```python
from build123d import *

# Parameters (mm, degrees)
SKETCH_1_W          = 55.5
SKETCH_1_H          = 46.5
EXTRUDE_1_DEPTH     = 15
SKETCH_2_W          = 6.5
SKETCH_2_H          = 6.5
CUT_EXTRUDE_1_DEPTH = 14
FILLET_1_R          = 2
SKETCH_3_W          = 4
SKETCH_3_H          = 34
EXTRUDE_2_DEPTH     = 5
SKETCH_4_W          = 55.5
SKETCH_4_H          = 46.5
EXTRUDE_3_DEPTH     = 1.5
SKETCH_5_R          = 1.5
CUT_EXTRUDE_2_DEPTH = 1
SKETCH_6_R          = 1.75
CUT_EXTRUDE_3_DEPTH = 2
SKETCH_7_W          = 33.995169083
SKETCH_7_H          = 13.97859025
SKETCH_7_W_2        = 5.219477383
SKETCH_7_H_2        = 24.424681599
SKETCH_7_W_3        = 25.720685112
SKETCH_7_H_3        = 6.003184014
EXTRUDE_4_DEPTH     = 10
SKETCH_8_W          = 33.995169083
SKETCH_8_H          = 13.97859025
SKETCH_8_W_2        = 25.720685112
SKETCH_8_H_2        = 6.003184014
CUT_EXTRUDE_4_DEPTH = 3
SKETCH_10_W         = 5.219477383
SKETCH_10_H         = 24.424681599
EXTRUDE_6_DEPTH     = 1.5


with BuildPart() as part:
    # 草图1 → 凸台-拉伸1 (new body)
    with BuildSketch(Plane.XY):
        Rectangle(SKETCH_1_W, SKETCH_1_H)
    extrude(amount=EXTRUDE_1_DEPTH)

    # 草图2 → 切除-拉伸1 (cut)
    with BuildSketch(Plane.XY.offset(15)):
        with Locations((-24.5, 20)):
            Rectangle(SKETCH_2_W, SKETCH_2_H)
        with Locations((24.5, 20)):
            Rectangle(SKETCH_2_W, SKETCH_2_H)
        with Locations((24.5, -20)):
            Rectangle(SKETCH_2_W, SKETCH_2_H)
        with Locations((-24.5, -20)):
            Rectangle(SKETCH_2_W, SKETCH_2_H)
    extrude(amount=-CUT_EXTRUDE_1_DEPTH, mode=Mode.SUBTRACT)

    # 圆角1
    fillet_1_edges = [part.edges().sort_by_distance(p)[0] for p in [
        (-21.25, 16.75, 8),
        (21.25, 16.75, 8),
        (21.25, -16.75, 8),
        (-21.25, -16.75, 8),
    ]]
    fillet(fillet_1_edges, radius=FILLET_1_R)

    # 草图3 → 凸台-拉伸2 (add)
    with BuildSketch(Plane.XY.offset(15)):
        with Locations((-18.75, 0.147123408)):
            Rectangle(SKETCH_3_W, SKETCH_3_H)
        with Locations((18.75, 0.147123408)):
            Rectangle(SKETCH_3_W, SKETCH_3_H)
    extrude(amount=EXTRUDE_2_DEPTH)

    # 草图4 → 凸台-拉伸3 (add)
    with BuildSketch(Plane.XY.offset(20)):
        Rectangle(SKETCH_4_W, SKETCH_4_H)
    extrude(amount=EXTRUDE_3_DEPTH)

    # 草图5 → 切除-拉伸2 (cut)
    with BuildSketch(Plane.XY.offset(1)):
        with Locations((24.5, 20)):
            Circle(SKETCH_5_R)
        with Locations((-24.5, 20)):
            Circle(SKETCH_5_R)
        with Locations((-24.5, -20)):
            Circle(SKETCH_5_R)
        with Locations((24.5, -20)):
            Circle(SKETCH_5_R)
    extrude(amount=-CUT_EXTRUDE_2_DEPTH, mode=Mode.SUBTRACT)

    # 草图6 → 切除-拉伸3 (cut)
    with BuildSketch(Plane.XY.offset(21.5)):
        with Locations((-24.5, 20)):
            Circle(SKETCH_6_R)
        with Locations((24.5, 20)):
            Circle(SKETCH_6_R)
        with Locations((24.5, -20)):
            Circle(SKETCH_6_R)
        with Locations((-24.5, -20)):
            Circle(SKETCH_6_R)
    extrude(amount=-CUT_EXTRUDE_3_DEPTH, mode=Mode.SUBTRACT)

    # 草图7 → 凸台-拉伸4 (add)
    with BuildSketch(Plane.XY.offset(21.5)):
        with Locations((0.947079491, 16.260704875)):
            Rectangle(SKETCH_7_W, SKETCH_7_H)
        with Locations((-25.140261309, -0.747694334)):
            Rectangle(SKETCH_7_W_2, SKETCH_7_H_2)
        with Locations((1.993851559, -20.248407993)):
            Rectangle(SKETCH_7_W_3, SKETCH_7_H_3)
    extrude(amount=EXTRUDE_4_DEPTH)

    # 草图8 → 切除-拉伸4 (cut)
    with BuildSketch(Plane.XY.offset(31.5)):
        with Locations((0.947079491, 16.260704875)):
            Rectangle(SKETCH_8_W, SKETCH_8_H)
        with Locations((1.993851559, -20.248407993)):
            Rectangle(SKETCH_8_W_2, SKETCH_8_H_2)
    extrude(amount=-CUT_EXTRUDE_4_DEPTH, mode=Mode.SUBTRACT)

    # 草图10 → 凸台-拉伸6 (add)
    with BuildSketch(Plane.XY.offset(31.5)):
        with Locations((-25.140261309, -0.747694334)):
            Rectangle(SKETCH_10_W, SKETCH_10_H)
    extrude(amount=EXTRUDE_6_DEPTH)


solid = part.part
```
Part model, mm, in its own coordinate system. A direction names the side the tool comes from. Round coordinates to 2 decimals unless told otherwise and drop trailing zeros. Order: outer loops, then holes, each group sorted by start corner. A loop starts at its lowest first (then second) coordinate and runs counter-clockwise, first axis right, second up. Notation, with made-up numbers: M 66.25,54.25 L 94.25,54.25 A18 cw 94.25,61.25 Z; hole C -10.5,12.5 d10. An arc over 180 degrees is marked long. Put each result on its own line as item: value. Start each with the question number.
1. Drop flat-ended pins along their axis: pin 1 (3.5 mm diameter, centred on x = -26, z = 8, fed in from -Y); pin 2 (1.5 mm diameter, centred on y = -10, z = 18.5, fed in from +X); pin 3 (1.3 mm diameter, centred on y = 21, z = 8, fed in from +X); pin 4 (10 mm diameter, centred on x = 20, y = 15, fed in from -Z). Give the stop position or say it passes through.
2. Two-plate mould, pull along X, no slides. Class faces 1 (the face through (23.39, -18.99, 0.51)), 2 (the face through (20.75, 0, 17)), 3 (the face through (-19, -16.853, 17)): +X half, -X half, draft (parallel to the pull), parting line (faces both ways), or undercut.
3. Slice it at D-D on y = 15. List the corners of the cut face in (x, z), then the cut area to 3 significant figures.
4. Slice it at B-B on z = 18. List the corners of the cut face in (x, y).
5. Drill centre lines: probe 1 along Y at (x, z) = (24.5, 0.55); probe 2 along Z at (x, y) = (-22.5, -20); probe 3 along Z at (x, y) = (-6.5, -2.5). Where is each one in solid material? Low to high. Write a range as [from, to].
6. Tool access for faces 4 (the face through (1, 9.271, 25)), 5 (the face through (-16.75, 0, 17)), 6 (the face through (21.25, -21, 8)): list every direction of +Z, -Z, +X, -X, +Y, -Y with a clear straight run to the whole face (end or side of a thin tool).
7. Slice it at C-C on y = 20. State how many separate pieces and enclosed holes the cut face has, then the cut area to 3 significant figures.
8. Slice it at A-A on x = -13.5. List the corners of the cut face in (y, z), then the cut area to 3 significant figures.
Findings:
1. pin 1: y = -16.75
1. pin 2: x = 20.75
1. pin 3: x = 21.25
1. pin 4: z = 0
2. face 1: undercut
2. face 2: +X half
2. face 3: draft
3. outline: M -27.75,0 L 27.75,0 L 27.75,15 L 20.75,15 L 20.75,20 L 27.75,20 L 27.75,21.5 L 17.94,21.5 L 17.94,28.5 L -16.05,28.5 L -16.05,21.5 L -27.75,21.5 L -27.75,20 L -20.75,20 L -20.75,15 L -27.75,15 Z; hole M -16.75,15 L 16.75,15 L 16.75,20 L -16.75,20 Z
3. area: 1,190 mm2
4. outline: M -20.75,-16.85 L -16.75,-16.85 L -16.75,17.15 L -20.75,17.15 Z; M 16.75,-16.85 L 20.75,-16.85 L 20.75,17.15 L 16.75,17.15 Z
5. probe 1: [-23.25, -21.5], [-18.5, 18.5], [21.5, 23.25]
5. probe 2: [0, 1], [20, 21.5]
5. probe 3: [0, 15], [20, 21.5]
6. face 4: +Z, +X
6. face 5: +Y, -Y
6. face 6: +X, -Y
7. separate pieces: 6
7. enclosed holes: 0
7. area: 955 mm2
8. outline: M -23.25,0 L 23.25,0 L 23.25,15 L -23.25,15 Z; M -23.25,20 L 23.25,20 L 23.25,28.5 L 9.27,28.5 L 9.27,21.5 L -23.25,21.5 Z
8. area: 865 mm2
